Source: CAD feature listing. Evaluate the final solid. Frame: model axes, mm. A direction names the side the tool comes from. Round coordinates to 2 decimals unless told otherwise and drop trailing zeros. Order: outer loops, then holes, each group sorted by start corner. A loop starts at its lowest first (then second) coordinate and runs counter-clockwise, first axis right, second up. Notation, with made-up numbers: M -1.5,48.5 L 40.5,48.5 A7 ccw 40.5,52.5 Z; hole C 36,-22.75 d10. An arc over 180 degrees is marked long. Answer as CSV lines item,"result". Start each with the question number.
Item 1: Section query D-D on y = 28. Return the cut outline in (x, z) (3 decimals), plus the area to 3 significant figures.
Item 2: Section query A-A on x = 0. Return the cut outline in (y, z) (3 decimals), plus the area to 3 significant figures.
Item 3: Set-up query: faces 1 (the face through (13, -13, 1.3)), 2 (the face through (1.67, -62.85, 8.35)), 3 (the face through (55.3, 29.91, 7.9)). Return all of +Z, -Z, +X, -X, +Y, -Y with unobstructed straight access to the full face (end or side cutting, diameter ignored); none if empty.
Item 4: Section query B-B on y = 0. Return the cut outline in (x, z) (3 decimals).
Item 5: First-contact query: P1, Ø1.5, axis at x = -25.5, z = 2.5, coming from the -Y side; P2, Ø1.5, axis at y = 21.5, z = 3.5, coming from the -X side; P3, Ø1, axis at y = -32.5, z = 6.5, coming from the +X side; P4, Ø20.5, axis at x = 0, y = 0, coming from the +Z side. Flat tips, straight axial feed; report the tip coordinate or a pass-through.
Item 6: Section query C-C on z = 3.25. Return the cut outline in (x, y), plus the area to 3 significant figures.
Item 7: Pull-direction query (X, two-part tool) for faces 4 (the face through (42, -47, 10.825)), 5 (the face through (-13.77, -61.99, 5.34)), 6 (the face through (-13.48, -60.72, 6)); classes: +X half, -X half, draft (parallel to the pull), parting line (faces both ways), or undercut.
Item 8: Line query: line 1 (Y direction, x = 0, z = 0.6); line 2 (Z direction, x = -12, y = 45); line 3 (Y direction, x = -42, z = 4.75). Output: solid intervals per line, ascending. Write a range as [from, to].
from build123d import *

# Parameters (mm, degrees)
F0_R      = 63.5
F1_DEPTH  = 1.3
F2_R      = 2.5
F3_DEPTH  = 25
F4_R      = 63.5
F4_R_2    = 62.2
F5_DEPTH  = 9.525
F7_R      = 1.75
F8_DEPTH  = 5
F9_COUNT  = 3
F11_R     = 17
F12_DEPTH = 25


with BuildPart() as f1:
    # F0 (on Top) → F1 (new body)
    with BuildSketch(Plane.XY):
        Circle(F0_R)
    extrude(amount=F1_DEPTH)

    # F2 (on face) → F3 (cut)
    with BuildSketch(Plane.XY.offset(1.3)):
        with Locations((-34.925, 0)):
            Circle(F2_R)
        with Locations((34.925, 0)):
            Circle(F2_R)
    extrude(amount=-F3_DEPTH, mode=Mode.SUBTRACT)

    # F4 (on face) → F5 (join)
    with BuildSketch(Plane.XY.offset(1.3)):
        Circle(F4_R)
        Circle(F4_R_2, mode=Mode.SUBTRACT)
    extrude(amount=F5_DEPTH)


with BuildPart() as f8:
    # F7 (on offset) → F8 (new body)
    with BuildSketch(Plane.XZ.offset(63.9)):
        with Locations((0, 7.825)):
            Circle(F7_R)
    extrude(amount=-F8_DEPTH)


with BuildPart() as f9_1:
    # F9: instance of F8
    add(f8.part.rotate(Axis((0, 0, 0), (0, 0, -1)), 1 * 360 / F9_COUNT))


with BuildPart() as f9_2:
    # F9: instance of F8
    add(f8.part.rotate(Axis((0, 0, 0), (0, 0, -1)), 2 * 360 / F9_COUNT))


with BuildPart() as f1_1:
    add(f1.part)

    # F10: cut F8, F9_2, F9_1
    add(f8.part, mode=Mode.SUBTRACT)
    add(f9_2.part, mode=Mode.SUBTRACT)
    add(f9_1.part, mode=Mode.SUBTRACT)

    # F11 (on face) → F12 (cut)
    with BuildSketch(Plane.XY.offset(1.3)):
        Circle(F11_R)
    extrude(amount=-F12_DEPTH, mode=Mode.SUBTRACT)


solid = f1_1.part
Results:
1,outline,"M -56.993,0 L 56.993,0 L 56.993,10.825 L 55.541,10.825 L 55.541,1.3 L -55.541,1.3 L -55.541,10.825 L -56.993,10.825 Z"
1,area,"176 mm^2"
2,outline,"M -63.5,0 L -17,0 L -17,1.3 L -62.2,1.3 L -62.2,6.075 L -63.5,6.075 Z; M -63.5,9.575 L -62.2,9.575 L -62.2,10.825 L -63.5,10.825 Z; M 17,0 L 63.5,0 L 63.5,10.825 L 62.2,10.825 L 62.2,1.3 L 17,1.3 Z"
2,area,"141 mm^2"
3,face 1,"+Z"
3,face 2,"-Y"
3,face 3,"none"
4,outline,"M -63.5,0 L -37.425,0 L -37.425,1.3 L -62.2,1.3 L -62.2,10.825 L -63.5,10.825 Z; M -32.425,0 L -17,0 L -17,1.3 L -32.425,1.3 Z; M 17,0 L 32.425,0 L 32.425,1.3 L 17,1.3 Z; M 37.425,0 L 63.5,0 L 63.5,10.825 L 62.2,10.825 L 62.2,1.3 L 37.425,1.3 Z"
5,P1,"y = -58.48"
5,P2,"x = -60.01"
5,P3,"x = 54.85"
5,P4,"through"
6,outline,"C 0,0 d127; hole C 0,0 d124.4"
6,area,"513 mm^2"
7,face 4,"draft"
7,face 5,"parting line"
7,face 6,"undercut"
8,line 1,"[-63.5, -17], [17, 63.5]"
8,line 2,"[0, 1.3]"
8,line 3,"[-47.63, -45.88], [45.88, 47.63]"
